Here's how the part is built. I have some questions about the finished solid (model axes, mm). Give positions to 0.01 mm unless a question says otherwise; leave off trailing zeros. Return JSON: item names as keys, results as strings. Group by question number.
(1) If we section it at A-A (y = 2.75): State how many separate pieces and enclosed holes the cut face has, then the cut area to 3 significant figures.
(2) For P1, Ø6, axis at x = 0, z = -51, coming from the -Y side; P2, Ø4, axis at y = 2, z = -2, coming from the +X side; P3, Ø3, axis at x = 35, z = 35, coming from the +Y side; P4, Ø5, axis at y = 7, z = 33, coming from the -X side, each with a flat end and sliding along its axis, tell me the tip position at first contact or that it passes through.
(3) If we mould it in two halves opening along Z, with no side actions, what happens to faces 1 (the flat face through (38, 8.6, -25)), 2 (the cylindrical face through (-0.96, 4.36, -48.69)), 3 (the cylindrical face through (56.133, 4.247, 12.465))? For each: released by +Z, released by -Z, zero draft, split by the parting line, or undercut.
(4) I need wall thicknesses on probe 1 along X at (y, z) = (5.25, 0); probe 2 along X at (y, z) = (3, -35); probe 3 along X at (y, z) = (7, -29). Which ranges of each line are inside material? Lowest first, please. Write a range as [from, to].
```python
from build123d import *

# Parameters (mm, degrees)
SKETCH_1_R          = 57.5
SKETCH_1_R_2        = 44.5
EXTRUDE_1_DEPTH     = 8.6
SKETCH_2_R          = 2.5
CUT_EXTRUDE_1_DEPTH = 82.770777176
CHAMFER_1_SIZE      = 0.5
SKETCH_3_R          = 1.65
CUT_EXTRUDE_2_DEPTH = 82.770777176


with BuildPart() as part:
    # ｽｹｯﾁ1 → ﾎﾞｽ - 押し出し1 (new body)
    with BuildSketch(Plane(origin=(0, 0, 0), x_dir=(1, 0, 0), z_dir=(0, 1, 0))):
        with Locations(Location((0, 0, 0), (0, 0, 90))):
            Circle(SKETCH_1_R)
        with Locations(Location((0, 0, 0), (0, 0, 90))):
            Circle(SKETCH_1_R_2, mode=Mode.SUBTRACT)
    extrude(amount=EXTRUDE_1_DEPTH)

    # ｽｹｯﾁ2 → ｶｯﾄ - 押し出し1 (cut, through all)
    with BuildSketch(Plane(origin=(0, 8.6, 0), x_dir=(1, 0, 0), z_dir=(0, 1, 0))):
        with Locations(Location((-51, 0, 0), (0, 0, 270))):
            Circle(SKETCH_2_R)
        with Locations(Location((0, 51, 0), (0, 0, 270))):
            Circle(SKETCH_2_R)
        with Locations(Location((51, 0, 0), (0, 0, 270))):
            Circle(SKETCH_2_R)
        with Locations(Location((0, -51, 0), (0, 0, 270))):
            Circle(SKETCH_2_R)
    extrude(amount=-CUT_EXTRUDE_1_DEPTH, mode=Mode.SUBTRACT)

    # 面取り1
    chamfer_1_edges = [part.edges().sort_by_distance(p)[0] for p in [
        (0, 0, 57.5),
        (0, 8.6, 57.5),
        (0, 0, 44.5),
        (0, 8.6, 44.5),
    ]]
    chamfer(chamfer_1_edges, length=CHAMFER_1_SIZE)

    # ｽｹｯﾁ3 → ｶｯﾄ - 押し出し2 (cut, through all)
    with BuildSketch(Plane(origin=(0, 8.6, 0), x_dir=(1, 0, 0), z_dir=(0, 1, 0))):
        with Locations(Location((-35, 35, 0), (0, 0, 270))):
            Circle(SKETCH_3_R)
        with Locations(Location((-35, -35, 0), (0, 0, 270))):
            Circle(SKETCH_3_R)
        with Locations(Location((35, -35, 0), (0, 0, 270))):
            Circle(SKETCH_3_R)
        with Locations(Location((35, 35, 0), (0, 0, 270))):
            Circle(SKETCH_3_R)
    extrude(amount=-CUT_EXTRUDE_2_DEPTH, mode=Mode.SUBTRACT)


solid = part.part
```
Values:
{
 "1": {"separate pieces": "1", "enclosed holes": "9", "area": "4,050 mm2"},
 "2": {"P1": "y = 0", "P2": "x = 57.5", "P3": "through", "P4": "x = -48.74"},
 "3": {"face 1": "zero draft", "face 2": "undercut", "face 3": "split by the parting line"},
 "4": {"probe 1": "[-57.5, -53.5], [-48.5, -44.5], [44.5, 48.5], [53.5, 57.5]", "probe 2": "[-45.62, -36.65], [-33.35, -27.48], [27.48, 33.35], [36.65, 45.62]", "probe 3": "[-49.65, -33.75], [33.75, 49.65]"}
}
